```python
from build123d import *

# Parameters (mm, degrees)
SKETCH1_W           = 203.2
SKETCH1_H           = 254
BOSS_EXTRUDE1_DEPTH = 3.175
FILLET1_R           = 25.4
SKETCH2_R           = 4
CUT_EXTRUDE1_DEPTH  = 25.4


with BuildPart() as part:
    # Sketch1 → Boss-Extrude1 (new body)
    with BuildSketch(Plane(origin=(0, 0, 0), x_dir=(1, 0, 0), z_dir=(0, 1, 0))):
        Rectangle(SKETCH1_W, SKETCH1_H)
    extrude(amount=BOSS_EXTRUDE1_DEPTH)

    # Fillet1
    fillet1_edges = [part.edges().sort_by_distance(p)[0] for p in [
        (101.6, 1.5875, 127),
        (-101.6, 1.5875, 127),
        (-101.6, 1.5875, -127),
        (101.6, 1.5875, -127),
    ]]
    fillet(fillet1_edges, radius=FILLET1_R)

    # Sketch2 → Cut-Extrude1 (cut)
    with BuildSketch(Plane.XZ):
        with Locations(Location((-79.1, 84.050000013, 0), (0, 0, 270))):
            Circle(SKETCH2_R)
        with Locations(Location((79.1, 84.050000013, 0), (0, 0, 270))):
            Circle(SKETCH2_R)
        with Locations(Location((79.1, -84.050000013, 0), (0, 0, 270))):
            Circle(SKETCH2_R)
        with Locations(Location((-79.1, -84.050000013, 0), (0, 0, 270))):
            Circle(SKETCH2_R)
    extrude(amount=-CUT_EXTRUDE1_DEPTH, mode=Mode.SUBTRACT)


solid = part.part
```
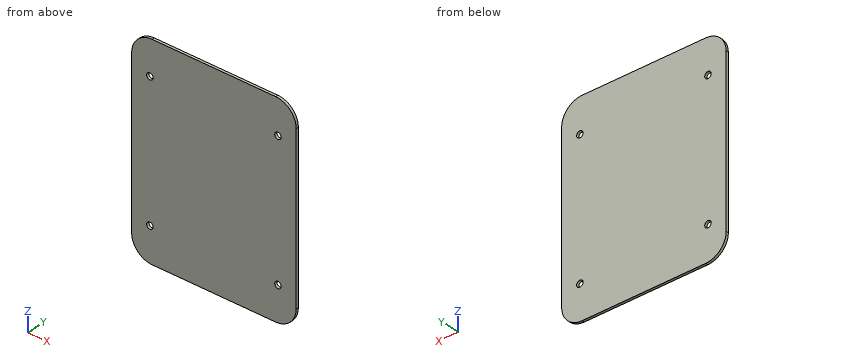
Check sheet for the modelled part. Datum: model origin and axes. Units: mm. Give positions to 0.01 mm unless a question says otherwise; leave off trailing zeros. Order: outer loops, then holes, each group sorted by start corner. A loop starts at its lowest first (then second) coordinate and runs counter-clockwise, first axis right, second up. Notation, with made-up numbers: (-14.5, 32.5) -> (44.5, 32.5) arc R7 ccw to (44.5, 43.5) -> close; hole circle Ø9 at (85, -37). An arc over 180 degrees is marked (long way). Return JSON: item names as keys, results as strings.
1. Cross-section at A-A, the plane z = -84.05. Record the cut outline in (x, y) (3 decimals), plus the area to 3 significant figures.
From the geometry:
{"outline": "(-101.6, 0) -> (-83.1, 0) -> (-83.1, 3.175) -> (-101.6, 3.175) -> close; (-75.1, 0) -> (75.1, 0) -> (75.1, 3.175) -> (-75.1, 3.175) -> close; (83.1, 0) -> (101.6, 0) -> (101.6, 3.175) -> (83.1, 3.175) -> close", "area": "594 mm^2"}
2. Cross-section at B-B, the plane x = 79.1. Record the cut outline in (y, z) (3 decimals), plus the area to 3 significant figures.
From the geometry:
{"outline": "(0, -126.834) -> (3.175, -126.834) -> (3.175, -88.05) -> (0, -88.05) -> close; (0, -80.05) -> (3.175, -80.05) -> (3.175, 80.05) -> (0, 80.05) -> close; (0, 88.05) -> (3.175, 88.05) -> (3.175, 126.834) -> (0, 126.834) -> close", "area": "755 mm^2"}
3. Cross-section at C-C, the plane x = -86. Record the cut outline in (y, z) (3 decimals).
From the geometry:
{"outline": "(0, -125.033) -> (3.175, -125.033) -> (3.175, 125.033) -> (0, 125.033) -> close"}
4. Material ranges on probe 1 along X at (y, z) = (2.05, -84.05); probe 2 along Z at (x, y) = (87.5, 1), recorded low to high. Write a range as [from, to].
From the geometry:
{"probe 1": "[-101.6, -83.1], [-75.1, 75.1], [83.1, 101.6]", "probe 2": "[-124.35, 124.35]"}
